Drawing for the job (mm, zero at the part's lowest x, y, z). Round coordinates to 2 decimals unless told otherwise and drop trailing zeros. Write each loop counter-clockwise with the first axis right and the second up, starting at its lowest first coordinate (ties: lowest second). Pieces come first, ordered by that corner, then holes.
Item 1: Band-saw the part on A-A, the plane y = 1. Write the cut outline in (x, z).
Item 2: Drop flat-ended pins along their axis: pin 1 Ø1.1 at (x, y) = (43, 6) entering from -Z; pin 2 Ø3 at (x, z) = (57.5, 21) entering from +Y; pin 3 Ø1.5 at (x, y) = (40.5, 6) entering from +Z. Give the stop position or say it passes through.
Item 3: Band-saw the part on C-C, the plane z = 65. Write the cut outline in (x, y).
Item 4: Wall check: probe 1 along Z at (x, y) = (43.5, 2.5); probe 2 along Y at (x, z) = (56, 27.5); probe 3 along X at (y, z) = (1, 34). Give the ranges that are in metal, low to high.
Item 5: Band-saw the part on B-B, the plane x = 52. Write the cut outline in (y, z).
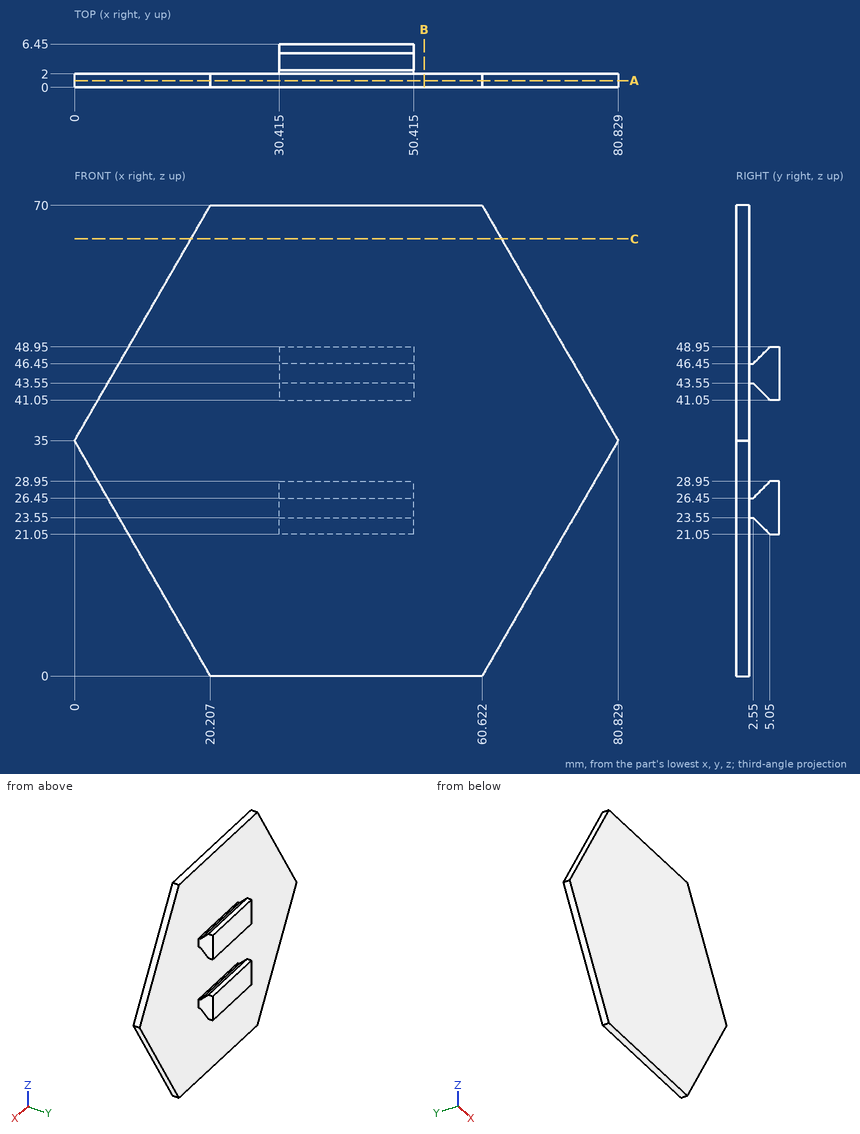
Results:
1. outline: (0, 35) - (20.21, 0) - (60.62, 0) - (80.83, 35) - (60.62, 70) - (20.21, 70) - close
2. pin 1: stops at z = 21.05
2. pin 2: stops at y = 2
2. pin 3: stops at z = 48.95
3. outline: (17.32, 0) - (63.51, 0) - (63.51, 2) - (17.32, 2) - close
4. probe 1: z = 23.55 to 26.45, 43.55 to 46.45
4. probe 2: y = 0 to 2
4. probe 3: x = 0.58 to 80.25
5. outline: (0, 0) - (2, 0) - (2, 70) - (0, 70) - close
